```python
from build123d import *

# Parameters (mm, degrees)
CROQUIS3_R              = 49
CROQUIS3_R_2            = 45
SALIENTE_EXTRUIR1_DEPTH = 56
CROQUIS1_R              = 77.574507489
SALIENTE_EXTRUIR2_DEPTH = 4
SALIENTE_EXTRUIR3_DEPTH = 38
CORTAR_EXTRUIR1_DEPTH   = 8
CROQUIS7_R              = 4
CORTAR_EXTRUIR2_DEPTH   = 42
REDONDEO1_R             = 4
REDONDEO2_R             = 1
CROQUIS8_R              = 1.3
CORTAR_EXTRUIR3_DEPTH   = 30.8


with BuildPart() as part:
    # Croquis3 → Saliente-Extruir1 (new body)
    with BuildSketch(Plane(origin=(0, 0, 0), x_dir=(1, 0, 0), z_dir=(0, 1, 0))):
        with Locations(Location((0, 0, 0), (0, 0, 270))):
            Circle(CROQUIS3_R)
        with Locations(Location((0, 0, 0), (0, 0, 270))):
            Circle(CROQUIS3_R_2, mode=Mode.SUBTRACT)
    extrude(amount=SALIENTE_EXTRUIR1_DEPTH)

    # Croquis1 → Saliente-Extruir2 (add)
    with BuildSketch(Plane(origin=(0, 0, 0), x_dir=(1, 0, 0), z_dir=(0, 1, 0))):
        with Locations(Location((0, 0, 0), (0, 0, 270))):
            Circle(CROQUIS1_R)
        with BuildLine():
            Line((-23.917575663, -38.117575663), (-10, -24.2))
            Line((-10, -24.2), (0, -24.2))
            Line((0, -24.2), (10, -24.2))
            Line((10, -24.2), (23.917575663, -38.117575663))
            ThreePointArc((23.917575663, -38.117575663), (12.444056717, -43.245178372), (0, -45))
            ThreePointArc((0, -45), (-6.760954384, -44.489206509), (-13.368422036, -42.968422036))
            ThreePointArc((-13.368422036, -42.968422036), (-15.776603613, -42.143786949), (-18.134305032, -41.184305032))
            ThreePointArc((-18.134305032, -41.184305032), (-21.081778264, -39.756240079), (-23.917575663, -38.117575663))
        make_face(mode=Mode.SUBTRACT)
        with BuildLine():
            Line((13.1, -15.2), (0, -15.2))
            Line((0, -15.2), (-13.1, -15.2))
            Line((-13.1, -15.2), (-30.752476319, -32.852476319))
            ThreePointArc((-30.752476319, -32.852476319), (-7.771708829, 44.323814613), (40.095012748, -20.430123659))
            ThreePointArc((40.095012748, -20.430123659), (37.628495356, -24.679877173), (34.713332708, -28.635372048))
            ThreePointArc((34.713332708, -28.635372048), (32.8007474, -30.807644668), (30.752476319, -32.852476319))
            Line((30.752476319, -32.852476319), (13.1, -15.2))
        make_face(mode=Mode.SUBTRACT)
    extrude(amount=SALIENTE_EXTRUIR2_DEPTH)

    # Croquis5 → Saliente-Extruir3 (add)
    with BuildSketch(Plane(origin=(0, 0, 0), x_dir=(1, 0, 0), z_dir=(0, 1, 0))):
        with BuildLine():
            ThreePointArc((18.658536585, 40.949469014), (14.835992877, 40.673601998), (13, 37.309516212))
            Line((13, 37.309516212), (13, 27.8))
            Line((13, 27.8), (0, 27.8))
            Line((0, 27.8), (-13, 27.8))
            Line((-13, 27.8), (-13, 37.309516212))
            ThreePointArc((-13, 37.309516212), (-14.835992877, 40.673601998), (-18.658536585, 40.949469014))
            ThreePointArc((-18.658536585, 40.949469014), (0, 45), (18.658536585, 40.949469014))
        make_face()
        Polygon((-13.1, -15.2), (13.1, -15.2), (13, -22.2), (-13.1, -22.2), align=None)
    extrude(amount=SALIENTE_EXTRUIR3_DEPTH)

    # Croquis6 → Cortar-Extruir1 (cut)
    with BuildSketch(Plane.XY.offset(15)):
        Polygon((5, 5), (0, 5), (-5, 5), (-5, 29), (-2.492829293, 29), (5, 29), align=None)
    extrude(amount=CORTAR_EXTRUIR1_DEPTH, mode=Mode.SUBTRACT)

    # Croquis7 → Cortar-Extruir2 (cut)
    with BuildSketch(Plane.XY.offset(15)):
        with Locations(Location((0, 12, 0), (0, 0, 180))):
            Circle(CROQUIS7_R)
    extrude(amount=CORTAR_EXTRUIR2_DEPTH, mode=Mode.SUBTRACT)

    # Redondeo1
    redondeo1_edges = [part.edges().sort_by_distance(p)[0] for p in [
        (0, 4, -49),
    ]]
    fillet(redondeo1_edges, radius=REDONDEO1_R)

    # Redondeo2
    # the kernel refuses this fillet: 1 mm, written as the material it adds along each edge
    with BuildSketch(Plane(origin=(-13.1, 4, 22.2), x_dir=(0, 0, 1), z_dir=(1, 0, 0))) as redondeo2_piece_1_section:
        with BuildLine():
            CenterArc((REDONDEO2_R, -REDONDEO2_R), REDONDEO2_R, 90, 90)
            Line((0, -REDONDEO2_R), (0, 0))
            Line((0, 0), (REDONDEO2_R, 0))
        make_face()
    redondeo2_piece_1 = extrude(amount=28.6, mode=Mode.PRIVATE)
    redondeo2_piece_1 = split(redondeo2_piece_1, bisect_by=Plane(origin=(12.992267362, 4.226395114, 22.741284648), z_dir=(-0.99989797479951, 0, -0.014284256782850096)), keep=Keep.TOP, mode=Mode.PRIVATE)
    add(redondeo2_piece_1)
    with BuildSketch(Plane(origin=(12.964289358, 4, 24.699744937), x_dir=(0.99989797479951, 0, 0.014284256782850096), z_dir=(0.014284256782850096, 0, -0.99989797479951))) as redondeo2_piece_2_section:
        with BuildLine():
            CenterArc((REDONDEO2_R, -REDONDEO2_R), REDONDEO2_R, 90, 90)
            Line((0, -REDONDEO2_R), (0, 0))
            Line((0, 0), (REDONDEO2_R, 0))
        make_face()
    redondeo2_piece_2 = extrude(amount=12.000714249, mode=Mode.PRIVATE)
    redondeo2_piece_2 = split(redondeo2_piece_2, bisect_by=Plane(origin=(14.988415496, 4.230359827, 17.088415496), z_dir=(-0.7071067811865411, 0, 0.7071067811865539)), keep=Keep.TOP, mode=Mode.PRIVATE)
    redondeo2_piece_2 = split(redondeo2_piece_2, bisect_by=Plane(origin=(13.268129446, 4.230359827, 15.2), z_dir=(0, 0, 1)), keep=Keep.TOP, mode=Mode.PRIVATE)
    redondeo2_piece_2 = split(redondeo2_piece_2, bisect_by=Plane(origin=(13.268129446, 4.230359827, 22.2), z_dir=(0, 0, -1)), keep=Keep.TOP, mode=Mode.PRIVATE)
    add(redondeo2_piece_2)
    with BuildSketch(Plane(origin=(-13.1, 4, 15.2), x_dir=(-1, 0, 0), z_dir=(0, 0, 1))) as redondeo2_piece_3_section:
        with BuildLine():
            CenterArc((REDONDEO2_R, -REDONDEO2_R), REDONDEO2_R, 90, 90)
            Line((0, -REDONDEO2_R), (0, 0))
            Line((0, 0), (REDONDEO2_R, 0))
        make_face()
    redondeo2_piece_3 = extrude(amount=7, mode=Mode.PRIVATE)
    redondeo2_piece_3 = split(redondeo2_piece_3, bisect_by=Plane(origin=(-15.014877598, 4.230417942, 17.114877598), z_dir=(0.7071067811865538, 0, 0.7071067811865414)), keep=Keep.TOP, mode=Mode.PRIVATE)
    add(redondeo2_piece_3)
    with BuildSketch(Plane(origin=(-13.1, 4, 15.2), x_dir=(-1, 0, 0), z_dir=(0, 0, 1))) as redondeo2_piece_4a_section:
        with BuildLine():
            CenterArc((REDONDEO2_R, -REDONDEO2_R), REDONDEO2_R, 90, 90)
            Line((0, -REDONDEO2_R), (0, 0))
            Line((0, 0), (REDONDEO2_R, 0))
        make_face()
    redondeo2_piece_4a = extrude(amount=9.5, mode=Mode.PRIVATE)
    redondeo2_piece_4a = split(redondeo2_piece_4a, bisect_by=Plane(origin=(-13.326395114, 4.226395114, 22.2), z_dir=(0, 0, 1)), keep=Keep.TOP, mode=Mode.PRIVATE)
    with BuildSketch(Plane(origin=(-15.6, 4, 22.2), x_dir=(0, 0, 1), z_dir=(1, 0, 0))) as redondeo2_piece_4b_section:
        with BuildLine():
            CenterArc((REDONDEO2_R, -REDONDEO2_R), REDONDEO2_R, 90, 90)
            Line((0, -REDONDEO2_R), (0, 0))
            Line((0, 0), (REDONDEO2_R, 0))
        make_face()
    redondeo2_piece_4b = extrude(amount=31.1, mode=Mode.PRIVATE)
    redondeo2_piece_4b = split(redondeo2_piece_4b, bisect_by=Plane(origin=(-13.1, 4.226395114, 22.426395114), z_dir=(-1, 0, 0)), keep=Keep.TOP, mode=Mode.PRIVATE)
    redondeo2_piece_4 = redondeo2_piece_4a & redondeo2_piece_4b
    add(redondeo2_piece_4)
    with BuildSketch(Plane(origin=(-13.1, 4, 22.2), x_dir=(0, 0, 1), z_dir=(1, 0, 0))) as redondeo2_piece_5a_section:
        with BuildLine():
            CenterArc((REDONDEO2_R, -REDONDEO2_R), REDONDEO2_R, 90, 90)
            Line((0, -REDONDEO2_R), (0, 0))
            Line((0, 0), (REDONDEO2_R, 0))
        make_face()
    redondeo2_piece_5a = extrude(amount=28.6, mode=Mode.PRIVATE)
    redondeo2_piece_5a = split(redondeo2_piece_5a, bisect_by=Plane(origin=(12.997017375, 4.226238422, 22.408783729), z_dir=(0.99989797479951, 0, 0.014284256782850096)), keep=Keep.TOP, mode=Mode.PRIVATE)
    with BuildSketch(Plane(origin=(12.964289358, 4, 24.699744937), x_dir=(0.99989797479951, 0, 0.014284256782850096), z_dir=(0.014284256782850096, 0, -0.99989797479951))) as redondeo2_piece_5b_section:
        with BuildLine():
            CenterArc((REDONDEO2_R, -REDONDEO2_R), REDONDEO2_R, 90, 90)
            Line((0, -REDONDEO2_R), (0, 0))
            Line((0, 0), (REDONDEO2_R, 0))
        make_face()
    redondeo2_piece_5b = extrude(amount=12.000714249, mode=Mode.PRIVATE)
    redondeo2_piece_5b = split(redondeo2_piece_5b, bisect_by=Plane(origin=(13.208805032, 4.226238422, 22.2), z_dir=(0, 0, 1)), keep=Keep.TOP, mode=Mode.PRIVATE)
    redondeo2_piece_5 = redondeo2_piece_5a & redondeo2_piece_5b
    add(redondeo2_piece_5)

    # Croquis8 → Cortar-Extruir3 (cut)
    with BuildSketch(Plane(origin=(0, 60, 0), x_dir=(1, 0, 0), z_dir=(0, 1, 0))):
        with Locations(Location((-5, -17.7, 0), (0, 0, 270))):
            Circle(CROQUIS8_R)
        with Locations(Location((5, -17.7, 0), (0, 0, 270))):
            Circle(CROQUIS8_R)
        with Locations(Location((5, 30.3, 0), (0, 0, 270))):
            Circle(CROQUIS8_R)
        with Locations(Location((-5, 30.3, 0), (0, 0, 270))):
            Circle(CROQUIS8_R)
    extrude(amount=-CORTAR_EXTRUIR3_DEPTH, mode=Mode.SUBTRACT)


solid = part.part
```
Build history of the part. All positions in model axes, mm. A direction names the side the tool comes from. Round coordinates to 2 decimals unless told otherwise and drop trailing zeros. Write each loop counter-clockwise with the first axis right and the second up, starting at its lowest first coordinate (ties: lowest second). Pieces come first, ordered by that corner, then holes. Notation, with made-up numbers: (42, 88) - (79, 88) arc R7 cw to (79, 100) - close; hole circle Ø1 at (84, 10.25). An arc over 180 degrees is marked (long way). Answer as CSV lines item,"result".
Q1. Cut at B-B (y = 12). Write the cut outline in (x, z), and give its area (3 significant figures).
Report:
outline,"(-18.66, -40.95) arc R45 cw to (-4, 44.82) - (-4, 48.84) arc R49 ccw (long way) to (4, 48.84) - (4, 44.82) arc R45 cw to (18.66, -40.95) arc R4 cw to (13, -37.31) - (13, -27.8) - (-13, -27.8) - (-13, -37.31) arc R4 cw to start; (-13.1, 15.2) - (-5, 15.2) - (-5, 22.2) - (-13.1, 22.2) - close; (5, 15.2) - (13.1, 15.2) - (13, 22.2) - (5, 22.2) - close"
area,"1,710 mm^2"
Q2. Drop flat-ended pins along their axis: pin 1 (2 mm diameter, centred on x = 5, z = -31, fed in from +Y); pin 2 (1.5 mm diameter, centred on x = -33.5, y = 22.5, fed in from -Z); pin 3 (10.5 mm diameter, centred on y = 28, z = -33.5, fed in from +X). Give the stop position or say it passes through.
Report:
pin 1,"stops at y = 38"
pin 2,"stops at z = -36.45"
pin 3,"stops at x = 40.04"
Q3. Pull direction Z, two halves, no side cores. Call faces 1 (the cylindrical face through (0.867, 15.905, 46.882)), 2 (the flat face through (0, 19, -27.8)), 3 (the cylindrical face through (14.718, 31.664, 46.737)): +Z half, -Z half, draft (parallel to the pull), parting line (faces both ways), or undercut.
Report:
face 1,"draft"
face 2,"undercut"
face 3,"parting line"
Q4. Cut at D-D (x = -62). Write the cut outline in (y, z).
Report:
outline,"(0, -46.62) - (4, -46.62) - (4, 46.62) - (0, 46.62) - close"
Q5. Tool access for faces 4 (the flat face through (6, 19, 15.2)), 5 (the flat face through (0, 38, -37)), 6 (the flat face through (0, 5, 19)): list every direction of +Z, -Z, +X, -X, +Y, -Y with a clear straight run to the whole face (end or side of a thin tool).
Report:
face 4,"+Y, -Y"
face 5,"+Y"
face 6,"none"
Q6. Cut at C-C (z = 61). Write the cut outline in (x, y).
Report:
outline,"(-47.92, 0) - (47.92, 0) - (47.92, 4) - (-47.92, 4) - close"
Q7. Cut at A-A (y = 31.5). Write the cut outline in (x, z).
Report:
outline,"circle Ø98 at (0, 0); (-13.1, 15.2) - (13.1, 15.2) - (13, 22.2) - (-13.1, 22.2) - close; hole (-18.66, -40.95) arc R4 ccw to (-13, -37.31) - (-13, -27.8) - (13, -27.8) - (13, -37.31) arc R4 ccw to (18.66, -40.95) arc R45 ccw (long way) to start; hole circle Ø2.6 at (-5, -30.3); hole circle Ø2.6 at (-5, 17.7); hole circle Ø2.6 at (5, -30.3); hole circle Ø2.6 at (5, 17.7)"
Q8. Drill centre lines: probe 1 along X at (y, z) = (34.5, 17.7); probe 2 along X at (y, z) = (31, 17); probe 3 along X at (y, z) = (43, 0). Where is each one in solid material? Low to high. Write a range as [from, to].
Report:
probe 1,"x = [-45.69, -41.37], [-13.1, -6.3], [-3.7, 3.7], [6.3, 13.06], [41.37, 45.69]"
probe 2,"x = [-45.96, -41.67], [-13.1, -6.1], [-3.9, 3.9], [6.1, 13.07], [41.67, 45.96]"
probe 3,"x = [-49, -45], [45, 49]"
